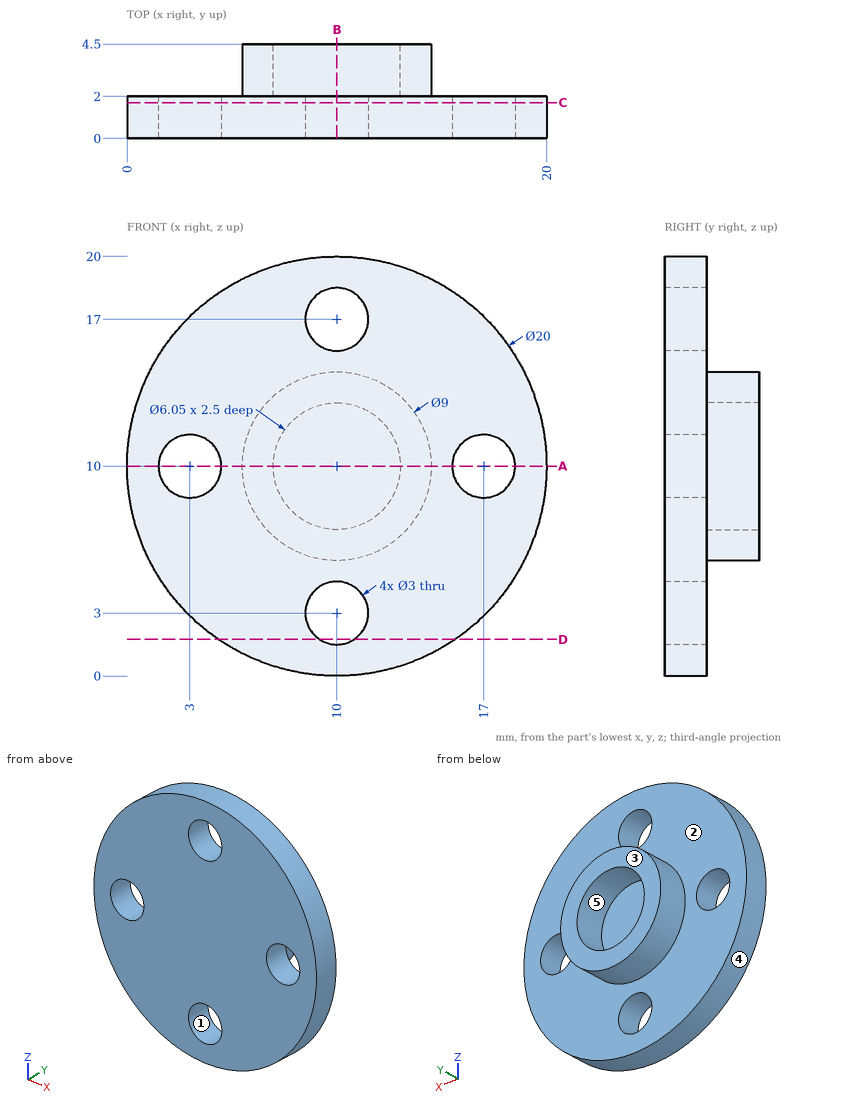
Geometry check sheet. Reference: drawing and pictorial views, mm from the part's lowest x, y, z. A direction names the side the tool comes from. Give positions to 0.01 mm unless a question says otherwise; leave off trailing zeros. Write each loop counter-clockwise with the first axis right and the second up, starting at its lowest first coordinate (ties: lowest second). Pieces come first, ordered by that corner, then holes.
Item 1: Cross-section at D-D (z = 1.75). Enter the section's corners in (x, y).
Item 2: Cross-section at A-A (z = 10). Enter the section's corners in (x, y) (3 decimals).
Item 3: Cross-section at B-B (x = 10). Enter the section's corners in (y, z) (3 decimals), and give its area (3 significant figures).
Item 4: Access from +Z, -Z, +X, -X, +Y, -Y to the whole of each face (thin tool, end or side, straight path). Record for the marked faces 1 and 2.
Item 5: Gauge pin test, flat ends, axial feed: pin 1 (1.5 mm diameter, centred on x = 5, y = 2, fed in from -Z); pin 2 (3 mm diameter, centred on x = 9, z = 9.5, fed in from +Y); pin 3 (2 mm diameter, centred on y = 1.5, z = 9, fed in from -X); pin 4 (2 mm diameter, centred on x = 15.5, y = 1.5, fed in from +Z). Record the tip position at first contact, or that the pin passes through.
Item 6: Scan lines: L1, parallel to X at y = 0.5, z = 10; L2, parallel to X at y = 2.65, z = 10 (3 decimals); L3, parallel to Z at x = 9.75, y = 0.2. Record each from-to range of solid material in increasing order.
Item 7: Draft check along Z on the marked faces 3, 4 and 5. Enter one of: released by +Z, released by -Z, zero draft, split by the parting line, or undercut.
Item 8: Cross-section at C-C (y = 1.7). Enter the section's corners in (x, z), and give its area (3 significant figures).
Report:
1. outline: (4.35, 0) - (9.17, 0) - (9.17, 2) - (4.35, 2) - close; (10.83, 0) - (15.65, 0) - (15.65, 2) - (10.83, 2) - close
2. outline: (0, 0) - (1.5, 0) - (1.5, 2) - (0, 2) - close; (4.5, 0) - (15.5, 0) - (15.5, 2) - (14.5, 2) - (14.5, 4.5) - (13.025, 4.5) - (13.025, 2) - (6.975, 2) - (6.975, 4.5) - (5.5, 4.5) - (5.5, 2) - (4.5, 2) - close; (18.5, 0) - (20, 0) - (20, 2) - (18.5, 2) - close
3. outline: (0, 0) - (2, 0) - (2, 1.5) - (0, 1.5) - close; (0, 4.5) - (2, 4.5) - (2, 5.5) - (4.5, 5.5) - (4.5, 6.975) - (2, 6.975) - (2, 13.025) - (4.5, 13.025) - (4.5, 14.5) - (2, 14.5) - (2, 15.5) - (0, 15.5) - close; (0, 18.5) - (2, 18.5) - (2, 20) - (0, 20) - close
3. area: 35.4 mm2
4. face 1: +Y, -Y
4. face 2: +Y
5. pin 1: stops at z = 0.95
5. pin 2: stops at y = 2
5. pin 3: stops at x = 0
5. pin 4: stops at z = 18.93
6. L1: x = 0 to 1.5, 4.5 to 15.5, 18.5 to 20
6. L2: x = 5.5 to 6.975, 13.025 to 14.5
6. L3: z = 0 to 1.52, 4.48 to 15.52, 18.48 to 20
7. face 3: zero draft
7. face 4: split by the parting line
7. face 5: undercut
8. outline: circle Ø20 at (10, 10); hole circle Ø3 at (3, 10); hole circle Ø3 at (10, 3); hole circle Ø3 at (10, 17); hole circle Ø3 at (17, 10)
8. area: 286 mm2
